Geometry check sheet. Reference: the model listing, model coordinates, mm. Face numbers are marked on the shaded views. Give positions to 0.01 mm unless a question says otherwise; leave off trailing zeros. Write each loop counter-clockwise with the first axis right and the second up, starting at its lowest first coordinate (ties: lowest second). Pieces come first, ordered by that corner, then holes. Notation, with made-up numbers: (76.5, -30) -> (119.5, -30) arc R20 cw to (119.5, 2) -> close; hole circle Ø11 at (14.5, -11.5). An arc over 180 degrees is marked (long way). Use a Markdown table: item, result. Add a question column.
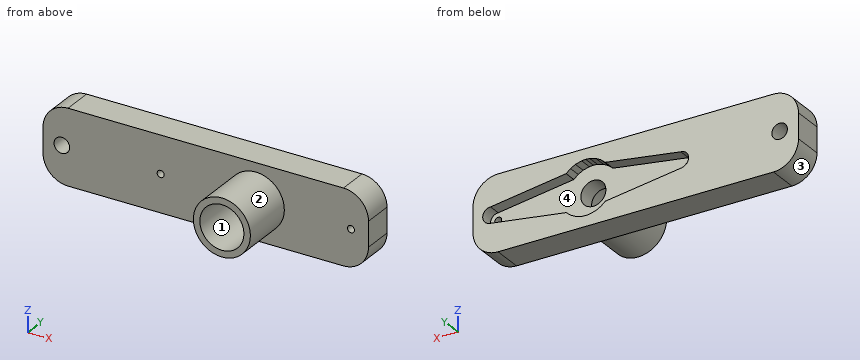
from build123d import *

# Parameters (mm, degrees)
ESQUISSE1_W             = 45
ESQUISSE1_H             = 15
BOSS_EXTRU_1_DEPTH      = 6
ESQUISSE2_R             = 2.5
ENL_V_MAT_EXTRU_1_DEPTH = 6
ESQUISSE4_R             = 0.7
ENL_V_MAT_EXTRU_2_DEPTH = 7
ENL_V_MAT_EXTRU_3_DEPTH = 2.5
ESQUISSE7_W             = 15
ESQUISSE7_H             = 6
BOSS_EXTRU_2_DEPTH      = 20
ESQUISSE8_R             = 1.55
ENL_V_MAT_EXTRU_4_DEPTH = 7.5
CONG_1_R                = 5
ESQUISSE9_R             = 5.693069504
ESQUISSE9_R_2           = 4.4
BOSS_EXTRU_3_DEPTH      = 11


with BuildPart() as part:
    # Esquisse1 → Boss.-Extru.1 (new body)
    with BuildSketch(Plane(origin=(0, 0, 0), x_dir=(1, 0, 0), z_dir=(0, 1, 0))):
        Rectangle(ESQUISSE1_W, ESQUISSE1_H)
    extrude(amount=BOSS_EXTRU_1_DEPTH)

    # Esquisse2 → Enlèv. mat.-Extru.1 (cut)
    with BuildSketch(Plane.XZ):
        with Locations(Location((0, 0, 0), (0, 0, 270))):
            Circle(ESQUISSE2_R)
    extrude(amount=-ENL_V_MAT_EXTRU_1_DEPTH, mode=Mode.SUBTRACT)

    # Esquisse4 → Enlèv. mat.-Extru.2 (cut)
    with BuildSketch(Plane.XZ):
        with Locations(Location((19, 0, 0), (0, 0, 270))):
            Circle(ESQUISSE4_R)
        with Locations(Location((-19, 0, 0), (0, 0, 270))):
            Circle(ESQUISSE4_R)
    extrude(amount=-ENL_V_MAT_EXTRU_2_DEPTH, mode=Mode.SUBTRACT)

    # Esquisse3 → Enlèv. mat.-Extru.3 (cut)
    with BuildSketch(Plane(origin=(0, 6, 0), x_dir=(1, 0, 0), z_dir=(0, 1, 0))):
        with BuildLine():
            Line((19, -1.561713939), (3.9, -3.75))
            Line((3.9, -3.75), (3.031885991, -4.483073583))
            Line((3.031885991, -4.483073583), (2.039673068, -5.012984659))
            Line((2.039673068, -5.012984659), (0.804642856, -5.351899783))
            Line((0.804642856, -5.351899783), (0, -5.41204965))
            Line((0, -5.41204965), (-0.804642856, -5.351899783))
            Line((-0.804642856, -5.351899783), (-2.039673068, -5.012984659))
            Line((-2.039673068, -5.012984659), (-3.031885991, -4.483073583))
            Line((-3.031885991, -4.483073583), (-3.9, -3.75))
            Line((-3.9, -3.75), (-19, -1.561713939))
            add(Edge.make_bspline(
                [(-19, -1.561713939), (-19.54064696, -1.574730153), (-20.339297961, -1.094989964), (-20.651707254, 0.047472401), (-20.293588536, 1.158800051), (-19.477708587, 1.555954085), (-19, 1.6)],
                knots=[0, 0, 0, 0, 0.329484693, 0.499358548, 0.699444054, 1, 1, 1, 1], degree=3))
            Line((-19, 1.6), (-3.9, 3.75))
            Line((-3.9, 3.75), (-3.031885991, 4.483073583))
            Line((-3.031885991, 4.483073583), (-2.039673068, 5.012984659))
            Line((-2.039673068, 5.012984659), (-0.804642856, 5.351899783))
            Line((-0.804642856, 5.351899783), (0, 5.41204965))
            Line((0, 5.41204965), (0.804642856, 5.351899783))
            Line((0.804642856, 5.351899783), (2.039673068, 5.012984659))
            Line((2.039673068, 5.012984659), (3.031885991, 4.483073583))
            Line((3.031885991, 4.483073583), (3.9, 3.75))
            Line((3.9, 3.75), (19, 1.6))
            add(Edge.make_bspline(
                [(19, -1.561713939), (19.54064696, -1.574730153), (20.339297961, -1.094989964), (20.651707254, 0.047472401), (20.293588536, 1.158800051), (19.477708587, 1.555954085), (19, 1.6)],
                knots=[0, 0, 0, 0, 0.329484693, 0.499358548, 0.699444054, 1, 1, 1, 1], degree=3))
        make_face()
    extrude(amount=-ENL_V_MAT_EXTRU_3_DEPTH, mode=Mode.SUBTRACT)

    # Esquisse7 → Boss.-Extru.2 (add)
    with BuildSketch(Plane.ZY.offset(22.5)):
        with Locations((0, 3)):
            Rectangle(ESQUISSE7_W, ESQUISSE7_H)
    extrude(amount=BOSS_EXTRU_2_DEPTH)

    # Esquisse8 → Enlèv. mat.-Extru.4 (cut)
    with BuildSketch(Plane.XZ):
        with Locations(Location((-38.739352064, 0, 0), (0, 0, 270))):
            Circle(ESQUISSE8_R)
    extrude(amount=-ENL_V_MAT_EXTRU_4_DEPTH, mode=Mode.SUBTRACT)

    # Congé1
    cong_1_edges = [part.edges().sort_by_distance(p)[0] for p in [
        (22.5, 3, 7.5),
        (22.5, 3, -7.5),
        (-42.5, 3, -7.5),
        (-42.5, 3, 7.5),
    ]]
    fillet(cong_1_edges, radius=CONG_1_R)

    # Esquisse9 → Boss.-Extru.3 (add)
    with BuildSketch(Plane.XZ):
        with Locations(Location((0, 0, 0), (0, 0, 270))):
            Circle(ESQUISSE9_R)
        with Locations(Location((0, 0, 0), (0, 0, 270))):
            Circle(ESQUISSE9_R_2, mode=Mode.SUBTRACT)
    extrude(amount=BOSS_EXTRU_3_DEPTH)


solid = part.part
1) Sectioned sample at D-D, the plane x = 13. Enter the section's corners in (y, z), and give its area (3 significant figures).
2) Sectioned sample at C-C, the plane y = 1.5. Enter the section's corners in (x, z), and give its area (3 significant figures).
3) Draft check along X on the marked faces 1, 2, 3 and 4. Enter one of: +X half, -X half, draft (parallel to the pull), parting line (faces both ways), or undercut.
4) Gauge pin test, flat ends, axial feed: P1, Ø2, axis at y = -7, z = 5, coming from the -X side; P2, Ø1.8, axis at x = -19, z = 0, coming from the +Y side; P3, Ø6.5, axis at x = 0, z = 0, coming from the -Y side. Record the tip position at first contact, or that the pin passes through.
5) Material ranges on probe 1 along X at (y, z) = (2.4, 0); probe 2 along Y at (x, z) = (-14, -4.75); probe 3 along X at (y, z) = (-6.75, 0), recorded low to high. Write a range as [from, to].
6) Sectioned sample at B-B, the plane z = 0. Count the separate pieces of the cut face and the enclosed holes in it, and give its area (3 significant figures).
7) Sectioned sample at A-A, the plane y = -5. Enter the section's corners in (x, z), and give its area (3 significant figures).
Check values:
| question | item | result |
|---|---|---|
| 1 | outline | (0, -7.5) -> (6, -7.5) -> (6, -2.45) -> (3.5, -2.45) -> (3.5, 2.43) -> (6, 2.43) -> (6, 7.5) -> (0, 7.5) -> close |
| 1 | area | 77.8 mm² |
| 2 | outline | (-42.5, -2.5) arc R5 ccw to (-37.5, -7.5) -> (17.5, -7.5) arc R5 ccw to (22.5, -2.5) -> (22.5, 2.5) arc R5 ccw to (17.5, 7.5) -> (-37.5, 7.5) arc R5 ccw to (-42.5, 2.5) -> close; hole circle Ø3.1 at (-38.74, 0); hole circle Ø1.4 at (-19, 0); hole circle Ø5 at (0, 0); hole circle Ø1.4 at (19, 0) |
| 2 | area | 923 mm² |
| 3 | face 1 | undercut |
| 3 | face 2 | parting line |
| 3 | face 3 | -X half |
| 3 | face 4 | undercut |
| 4 | P1 | x = -4.05 |
| 4 | P2 | y = 3.5 |
| 4 | P3 | y = 0 |
| 5 | probe 1 | [-42.5, -40.29], [-37.19, -19.7], [-18.3, -2.5], [2.5, 18.3], [19.7, 22.5] |
| 5 | probe 2 | [0, 6] |
| 5 | probe 3 | [-5.69, -4.4], [4.4, 5.69] |
| 6 | separate pieces | 5 |
| 6 | enclosed holes | 0 |
| 6 | area | 270 mm² |
| 7 | outline | circle Ø11.39 at (0, 0); hole circle Ø8.8 at (0, 0) |
| 7 | area | 41.0 mm² |
